Design review of the part shown in the three views and the two pictorial views. Dimensions are in mm from the part's minimum x, y and z. A direction names the side the tool comes from. Coordinates: 2 decimals unless noted, no trailing zeros. Loops run counter-clockwise (first coordinate to the right, second up) from the corner with the lowest first, then second, coordinate; pieces in that order, holes last.
Q1. Machinability: for the marked faces 1 and 2, which of the approach directions +Z, -Z, +X, -X, +Y, -Y give a long, thin tool a straight path to every point of the face, cutting with its end or side? Answer none if there is none.
Q2. Add section D-D on z = 157. Give the boundary of the cut face in (x, y), and give its area (3 significant figures).
Q3. Wall thickness on probe 1 along X at (y, z) = (66, 23); probe 2 along Z at (x, y) = (81, 66); probe 3 along X at (y, z) = (40, 26): over which ranges is each line inside the solid? List them lowest first.
Q4. Add section A-A on x = 86.5. Give the boundary of the cut face in (y, z) (3 decimals).
Q5. Add section B-B on y = 6. Give the boundary of the cut face in (x, z).
Q6. Draft analysis for pull direction X (two halves, no side actions). For the marked faces 3, 4, 5 and 6, state which applies: released by +X, released by -X, zero draft, split by the parting line, or undercut.
Q7. For P1, Ø5.5, axis at y = 66.5, z = 174.5, coming from the -X side; P2, Ø2.5, axis at x = 3, y = 40.5, coming from the +Z side; P3, Ø1.5, axis at y = 41.5, z = 174, coming from the -X side, all flat-tipped, find the tip position at first contact; note any pin that passes through.
Q8. Add section C-C on x = 116. Give the boundary of the cut face in (y, z), and give its area (3 significant figures).
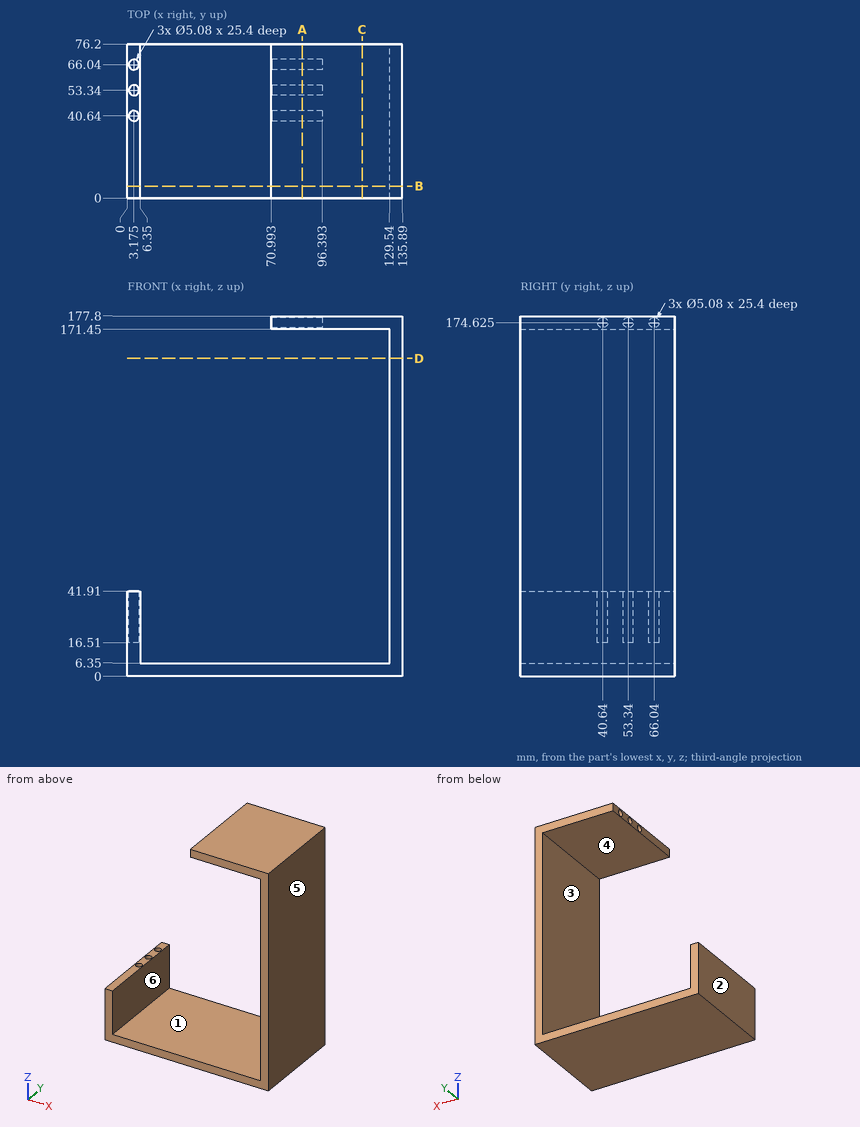
Entries:
1. face 1: +Y, -Y
1. face 2: +Z, -Z, -X, +Y, -Y
2. outline: (129.54, 0) - (135.89, 0) - (135.89, 76.2) - (129.54, 76.2) - close
2. area: 484 mm2
3. probe 1: x = 0 to 0.64, 5.71 to 6.35, 129.54 to 135.89
3. probe 2: z = 0 to 6.35, 171.45 to 172.09, 177.16 to 177.8
3. probe 3: x = 0 to 0.72, 5.63 to 6.35, 129.54 to 135.89
4. outline: (0, 0) - (76.2, 0) - (76.2, 6.35) - (0, 6.35) - close; (0, 171.45) - (76.2, 171.45) - (76.2, 177.8) - (0, 177.8) - close; hole circle Ø5.08 at (40.64, 174.625); hole circle Ø5.08 at (53.34, 174.625); hole circle Ø5.08 at (66.04, 174.625)
5. outline: (0, 0) - (135.89, 0) - (135.89, 177.8) - (70.99, 177.8) - (70.99, 171.45) - (129.54, 171.45) - (129.54, 6.35) - (6.35, 6.35) - (6.35, 41.91) - (0, 41.91) - close
6. face 3: undercut
6. face 4: zero draft
6. face 5: released by +X
6. face 6: undercut
7. P1: stops at x = 70.99
7. P2: stops at z = 16.51
7. P3: stops at x = 96.39
8. outline: (0, 0) - (76.2, 0) - (76.2, 6.35) - (0, 6.35) - close; (0, 171.45) - (76.2, 171.45) - (76.2, 177.8) - (0, 177.8) - close
8. area: 968 mm2
